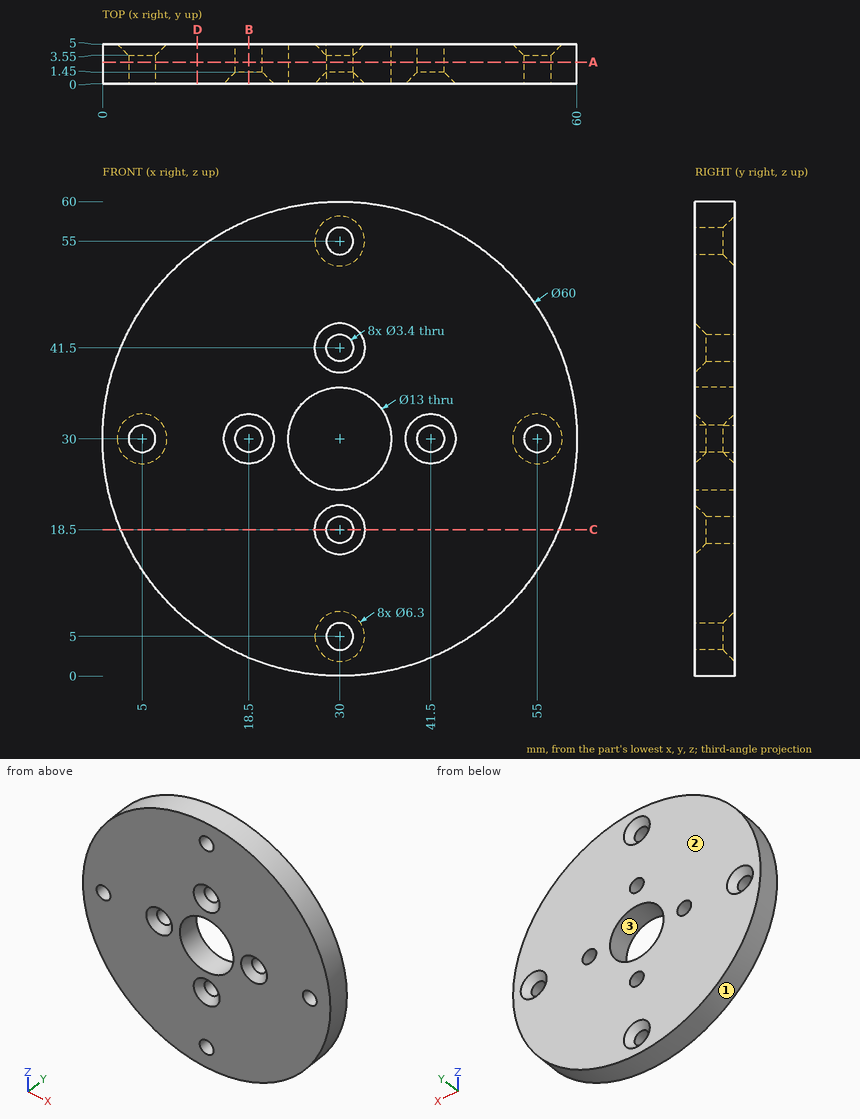
Study the drawing (mm; zero at the part's minimum x, y, z) and answer. Give positions to 0.01 mm unless a question says otherwise; leave off trailing zeros. Loops run counter-clockwise (first coordinate to the right, second up) from the corner with the lowest first, then second, coordinate; pieces in that order, holes last. Notation, with made-up numbers: (41.25, 34.5) - (61.25, 34.5) arc R20 ccw to (61.25, 51.5) - close; hole circle Ø5 at (30, 72). An arc over 180 degrees is marked (long way). Answer in a Markdown table with one row per item. Add a question column.
Q1. The part is cut by section A-A (y = 2.7). State how many separate pieces and enclosed holes the cut face has, and give its area (3 significant figures).
Q2. Each of these flat-tipped pins is pushed along its axis until it touches: P1, Ø1, axis at x = 21, y = 1, coming from the +Z side; P2, Ø3, axis at x = 18.5, z = 30, coming from the -Y side; P3, Ø3, axis at x = 54, y = 2, coming from the -Z side; P4, Ø1, axis at y = 1, z = 46, coming from the +X side. Where does it stop, or does it pass through?
Q3. The part is cut by section C-C (z = 18.5). Determine the outline of the cut face in (x, y).
Q4. Determine the mould class of the marked faces 1, 2 and 3 for opening direction Z: released by +Z, released by -Z, zero draft, split by the parting line, or undercut.
Q5. The part is cut by section D-D (x = 12). Determine the outline of the cut face in (y, z), and give its area (3 significant figures).
Q6. The part is cut by section B-B (x = 18.5). Determine the outline of the cut face in (y, z).
Q7. Consider line 1 along Z through (x, y) = (30, 2.25); line 2 along Z through (x, y) = (3.5, 3.8). Determine where each line is inside the solid, lowest interval first.
Solution:
| question | item | result |
|---|---|---|
| 1 | separate pieces | 1 |
| 1 | enclosed holes | 9 |
| 1 | area | 2,620 mm² |
| 2 | P1 | stops at z = 58.77 |
| 2 | P2 | passes through |
| 2 | P3 | stops at z = 10.16 |
| 2 | P4 | stops at x = 55.69 |
| 3 | outline | (2.29, 0) - (26.85, 0) - (28.3, 1.45) - (28.3, 5) - (2.29, 5) - close; (31.7, 1.45) - (33.15, 0) - (57.71, 0) - (57.71, 5) - (31.7, 5) - close |
| 4 | face 1 | split by the parting line |
| 4 | face 2 | zero draft |
| 4 | face 3 | undercut |
| 5 | outline | (0, 6) - (5, 6) - (5, 54) - (0, 54) - close |
| 5 | area | 240 mm² |
| 6 | outline | (0, 2.29) - (5, 2.29) - (5, 28.3) - (1.45, 28.3) - (0, 26.85) - close; (0, 33.15) - (1.45, 31.7) - (5, 31.7) - (5, 57.71) - (0, 57.71) - close |
| 7 | line 1 | z = 0 to 3.3, 6.7 to 16.8, 20.2 to 23.5, 36.5 to 39.8, 43.2 to 53.3, 56.7 to 60 |
| 7 | line 2 | z = 15.94 to 28.75, 31.25 to 44.06 |
